```python
from build123d import *

# Parameters (mm, degrees)
F0_W     = 80
F0_H     = 80
F1_DEPTH = 80
F2_R     = 7.5
F3_DEPTH = 5
F4_W     = 30
F4_H     = 15
F5_DEPTH = 5


with BuildPart() as f1:
    # F0 (on Top) → F1 (new body)
    with BuildSketch(Plane.XY):
        Rectangle(F0_W, F0_H)
    extrude(amount=F1_DEPTH)

    # F2 (on face) → F3 (join)
    with BuildSketch(Plane.XZ.offset(40)):
        with Locations((-20, 40)):
            Circle(F2_R)
        with Locations((20, 40)):
            Circle(F2_R)
    extrude(amount=F3_DEPTH)

    # F4 (on face) → F5 (cut)
    with BuildSketch(Plane.XZ.offset(40)):
        with Locations((0, 15)):
            Rectangle(F4_W, F4_H)
    extrude(amount=-F5_DEPTH, mode=Mode.SUBTRACT)


solid = f1.part
```
Work out the finished part from the listing and answer in its coordinate system (mm). A direction names the side the tool comes from. Round coordinates to 2 decimals unless told otherwise and drop trailing zeros. Write each loop counter-clockwise with the first axis right and the second up, starting at its lowest first coordinate (ties: lowest second). Pieces come first, ordered by that corner, then holes.
1) Flat-ended cylindrical pins translate along their axes: P1, Ø7.5, axis at x = 3, z = 16, coming from the -Y side; P2, Ø5, axis at x = 2, z = 50.5, coming from the -Y side. Find the tip coordinate at first contact, or state that the pin passes through.
2) Determine the mould class of faces 1 (the face through (-40, -1, 39)), 2 (the face through (0, -35, 15)), 3 (the face through (18.37, -42.46, 32.68)) for opening direction Z: pulls with the +Z half, pulls with the -Z half, needs draft (parallel to the pull), parting line crosses it, or undercut.
3) A cutting plane is placed at C-C on x = 20. Determine the outline of the cut face in (y, z).
4) A cutting plane is placed at B-B on x = 10.5. Determine the outline of the cut face in (y, z).
5) Which of the six approach directions +Z, -Z, +X, -X, +Y, -Y give full straight-line access (tool end or side, diameter ignored) to faces 4 (the face through (-1, 1, 0)), 5 (the face through (0, -38, 22.5))?
6) Consider probe 1 along Y at (x, z) = (32.5, 76); probe 2 along Y at (x, z) = (-9, 10.5). Determine where each line is inside the solid, lowest interval first.
7) A cutting plane is placed at A-A on z = 35.5. Determine the outline of the cut face in (x, y).
Entries:
1. P1: stops at y = -35
1. P2: stops at y = -40
2. face 1: needs draft
2. face 2: undercut
2. face 3: parting line crosses it
3. outline: (-45, 32.5) - (-40, 32.5) - (-40, 0) - (40, 0) - (40, 80) - (-40, 80) - (-40, 47.5) - (-45, 47.5) - close
4. outline: (-40, 0) - (40, 0) - (40, 80) - (-40, 80) - (-40, 22.5) - (-35, 22.5) - (-35, 7.5) - (-40, 7.5) - close
5. face 4: -Z, +X, -X, +Y, -Y
5. face 5: -Y
6. probe 1: y = -40 to 40
6. probe 2: y = -35 to 40
7. outline: (-40, -40) - (-26, -40) - (-26, -45) - (-14, -45) - (-14, -40) - (14, -40) - (14, -45) - (26, -45) - (26, -40) - (40, -40) - (40, 40) - (-40, 40) - close
